Input: part model. Units: mm. Frame: model coordinates. Face numbers are marked on the shaded views. A direction names the side the tool comes from. Round coordinates to 2 decimals unless told otherwise and drop trailing zeros. Loops run counter-clockwise (first coordinate to the right, second up) from the corner with the lowest first, then second, coordinate; pieces in that order, holes last.
(1) Access query for the marked faces 1, 2 and 3. Directions: +Z, -Z, +X, -X, +Y, -Y. A direction counts if a zero-diameter tool reaches every point of the face in a straight line with its end or side. Return the directions, or none.
(2) Cut plane B-B, the plane y = -9. Output: boundary loops of the cut face in (x, z).
(3) First-contact query: pin 1 Ø2 at (y, z) = (-49.5, 3.5) entering from -X; pin 2 Ø3 at (x, z) = (-5, 1.5) entering from +Y; pin 3 Ø1.5 at (y, z) = (17.5, 5.5) entering from -X; pin 4 Ø1.5 at (y, z) = (-4.5, 2.5) entering from -X. Flat tips, straight axial feed; report the tip coordinate or a pass-through.
(4) Line query: line 1 (Z direction, x = -33.5, y = 50); line 2 (X direction, y = 42, z = 0.75); line 3 (X direction, y = -22.5, z = 1). Output: solid intervals per line, ascending.
(5) Cut plane A-A, the plane x = 5. Output: boundary loops of the cut face in (y, z), and give its area (3 significant figures).
from build123d import *

# Parameters (mm, degrees)
PAD_DEPTH    = 7
SKETCH001_R  = 1.55
POCKET_DEPTH = 74.501
FILLET_R     = 3.4999
FILLET001_R  = 5


with BuildPart() as part:
    # Sketch → Pad (new body)
    with BuildSketch(Plane.XY):
        Polygon((-37.25, 35.794964), (-37.25, 53.5), (-30.25, 53.5), (-30.25, 38.5), (37.25, -35.794964), (37.25, -53.5), (30.25, -53.5), (30.25, -38.5), align=None)
    extrude(amount=PAD_DEPTH)

    # Sketch001 (on Face1 of Pad) → Pocket (cut, through all)
    with BuildSketch(Plane(origin=(-37.25, 0, 0), x_dir=(0, -1, 0), z_dir=(-1, 0, 0))):
        with Locations((-50, 3.5)):
            Circle(SKETCH001_R)
        with Locations((50, 3.5)):
            Circle(SKETCH001_R)
    extrude(amount=-POCKET_DEPTH, mode=Mode.SUBTRACT)

    # Fillet
    fillet_edges = [part.edges().sort_by_distance(p)[0] for p in [
        (-33.75, 53.5, 7),
        (-33.75, 53.5, 0),
        (33.75, -53.5, 0),
        (33.75, -53.5, 7),
    ]]
    fillet(fillet_edges, radius=FILLET_R)

    # Fillet001
    fillet001_edges = [part.edges().sort_by_distance(p)[0] for p in [
        (37.25, -35.794964, 3.5),
        (-30.25, 38.5, 3.5),
        (30.25, -38.5, 3.5),
        (-37.25, 35.794964, 3.5),
    ]]
    fillet(fillet001_edges, radius=FILLET001_R)


solid = part.part
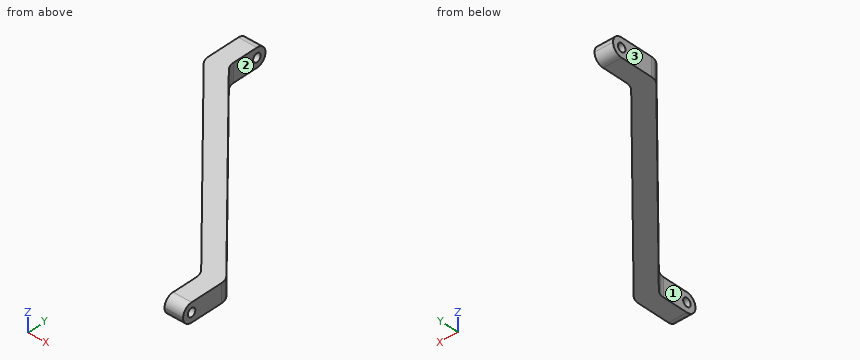
Reported:
1. face 1: +Z, -Z, -X, -Y
1. face 2: +Z, -Z, +X, +Y
1. face 3: +Z, -Z, -X, +Y, -Y
2. outline: (3.45, 0) - (12.91, 0) - (12.91, 7) - (3.45, 7) - close
3. pin 1: passes through
3. pin 2: stops at y = 12.36
3. pin 3: stops at x = -21.31
3. pin 4: stops at x = -1.32
4. line 1: z = 0 to 1.95, 5.05 to 7
4. line 2: x = -37.25 to -30.25
4. line 3: x = 15.71 to 25.17
5. outline: (-10.71, 0) - (-0.3, 0) - (-0.3, 7) - (-10.71, 7) - close
5. area: 72.9 mm2
